Source: three-view drawing plus pictorial views. Frame: mm from the lowest corner of the part. Coordinates: 2 decimals unless noted, no trailing zeros. Order: outer loops, then holes, each group sorted by start corner. A loop starts at its lowest first (then second) coordinate and runs counter-clockwise, first axis right, second up. Notation, with made-up numbers: (5, 46.5) - (62, 46.5) arc R5 cw to (62, 55.5) - close; hole circle Ø6 at (-5.5, 60.5). An arc over 180 degrees is marked (long way). One line per question, with ' | ' between items.
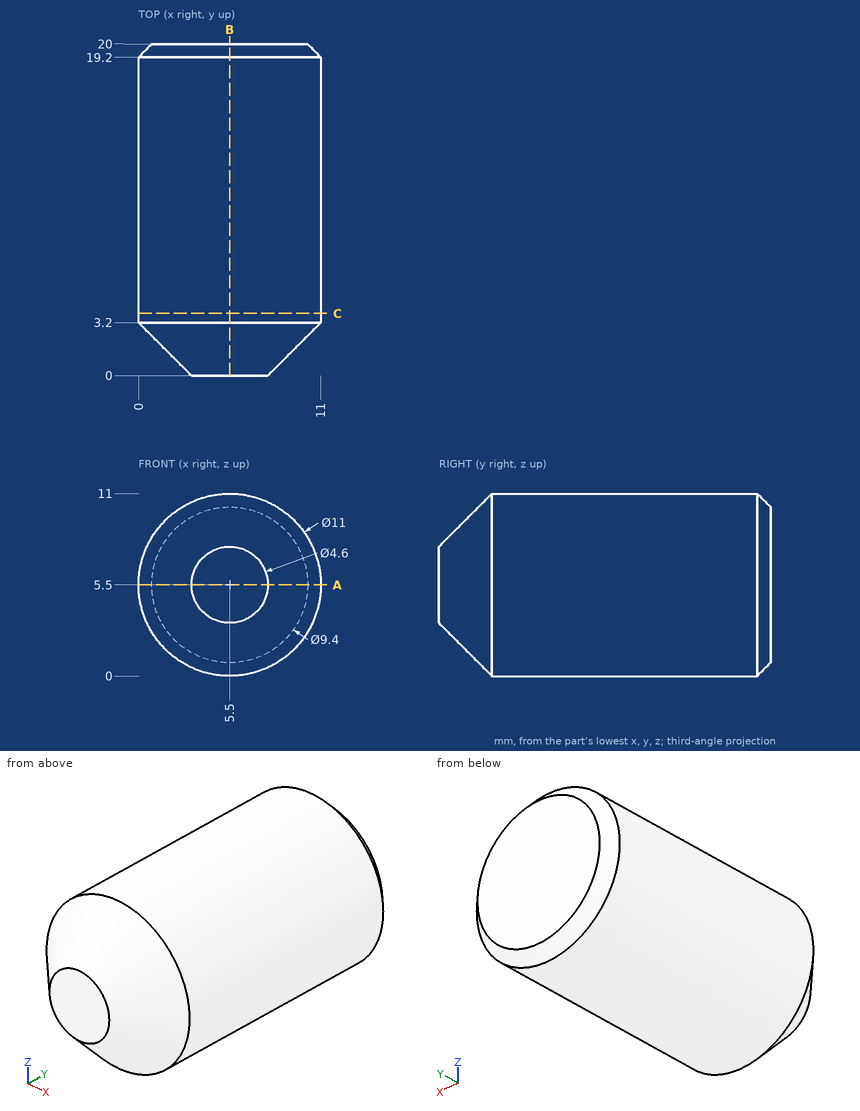
Item 1: Section B-B on x = 5.5. Return the cut outline in (y, z).
Data:
outline: (0, 3.2) - (3.2, 0) - (19.2, 0) - (20, 0.8) - (20, 10.2) - (19.2, 11) - (3.2, 11) - (0, 7.8) - close
Item 2: Section C-C on y = 3.75. Return the cut outline in (x, z), and give its area (3 significant figures).
Data:
outline: circle Ø11 at (5.5, 5.5) | area: 95.0 mm^2
Item 3: Section A-A on z = 5.5. Return the cut outline in (x, y), and give its area (3 significant figures).
Data:
outline: (0, 3.2) - (3.2, 0) - (7.8, 0) - (11, 3.2) - (11, 19.2) - (10.2, 20) - (0.8, 20) - (0, 19.2) - close | area: 209 mm^2
Item 4: Ray query, line 1 (Z direction, x = 8, y = 12); line 2 (X direction, y = 11.75, z = 2); line 3 (X direction, y = 12.25, z = 5.75). Return the intervals inside material, ascending.
Data:
line 1: 0.6 to 10.4 | line 2: 1.26 to 9.74 | line 3: 0.01 to 10.99
Item 5: Contact query for flat-ended pins moving along their axis: P1, Ø1, axis at x = 5, z = 9, coming from the -Y side; P2, Ø1.5, axis at x = 3, y = 7.5, coming from the +Z side; P3, Ø6, axis at y = 4.5, z = 2, coming from the +X side. Output: stop coordinate, or through.
Data:
P1: y = 0.74 | P2: z = 10.71 | P3: x = 10.98
